The drawing under review shows one solid part. Ordinate dimensions are in mm from its lowest x, y, z. A direction names the side the tool comes from. Give positions to 0.01 mm unless a question says otherwise; leave off trailing zeros. Write each loop counter-clockwise with the first axis right and the second up, starting at its lowest first coordinate (ties: lowest second). Pieces come first, ordered by that corner, then holes. Notation, with made-up numbers: M -14.5,35 L -9.5,35 A29 cw -9.5,62 Z; hole C 71,56.25 d7. An arc over 180 degrees is marked long. One line per item, written item: value. Start each with the question number.
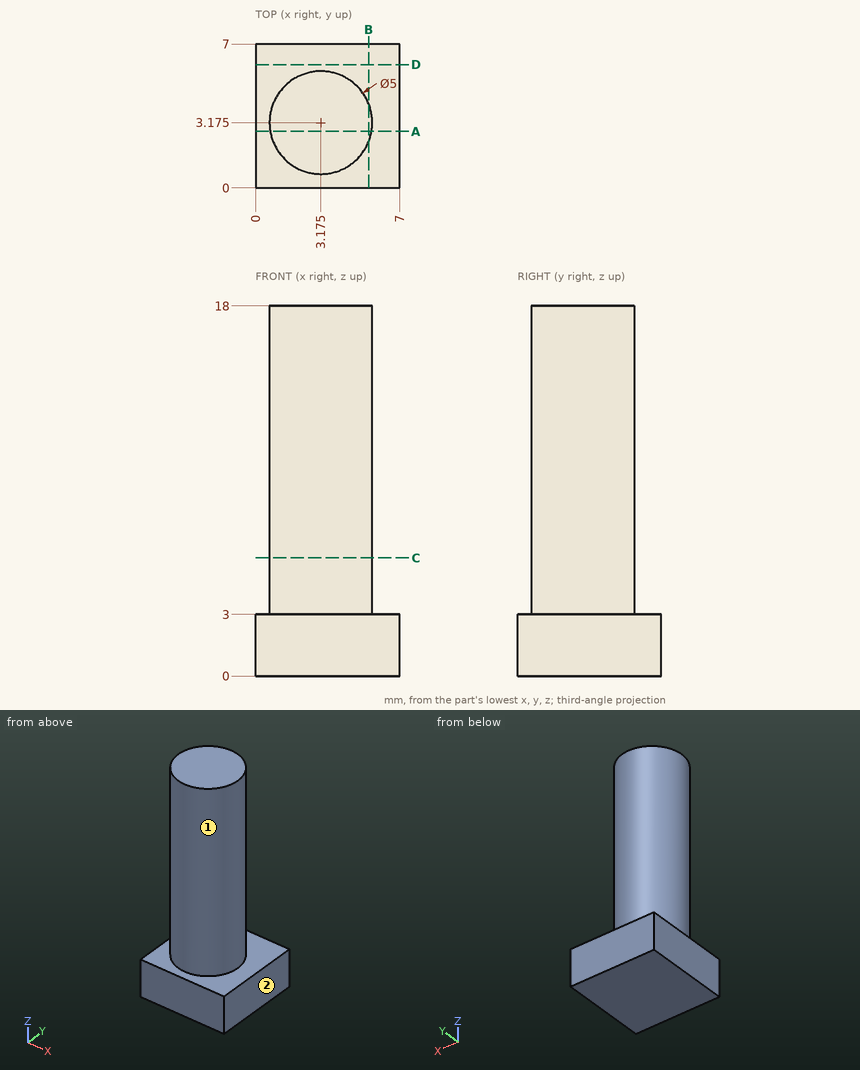
Q1. Take a section at A-A, the plane y = 2.75. Give the boundary of the cut face in (x, z).
Q2. Take a section at B-B, the plane x = 5.5. Give the boundary of the cut face in (y, z), then the cut area to 3 significant figures.
Q3. For P1, Ø2, axis at x = 3, z = 15.5, coming from the -Y side (3 decimals); P2, Ø4, axis at x = 2.5, z = 14.5, coming from the +Y side (3 decimals); P3, Ø4, axis at x = 3, y = 3.5, coming from the -Z side, all flat-tipped, find the tip position at first contact; note any pin that passes through.
Q4. Take a section at D-D, the plane y = 6. Give the boundary of the cut face in (x, z).
Q5. Wall thickness on line 1 (Z direction, x = 0.5, y = 6.5); line 2 (X direction, y = 3.25, z = 5.25); line 3 (Y direction, x = 2.5, z = 8.5): over which ranges is each line inside the solid? List them lowest first. Write a range as from..to.
Q6. Take a section at C-C, the plane z = 5.75. Give the boundary of the cut face in (x, y) (3 decimals), then the cut area to 3 significant figures.
Q7. Machinability: for the marked faces 1 and 2, which of the approach directions +Z, -Z, +X, -X, +Y, -Y give a long, thin tool a straight path to every point of the face, cutting with its end or side? Answer none if there is none.
Results list:
1. outline: M 0,0 L 7,0 L 7,3 L 5.64,3 L 5.64,18 L 0.71,18 L 0.71,3 L 0,3 Z
2. outline: M 0,0 L 7,0 L 7,3 L 4.09,3 L 4.09,18 L 2.26,18 L 2.26,3 L 0,3 Z
2. area: 48.6 mm^2
3. P1: stops at y = 0.675
3. P2: stops at y = 5.675
3. P3: stops at z = 0
4. outline: M 0,0 L 7,0 L 7,3 L 0,3 Z
5. line 1: z = 0..3
5. line 2: x = 0.68..5.67
5. line 3: y = 0.77..5.58
6. outline: C 3.175,3.175 d5
6. area: 19.6 mm^2
7. face 1: +Z
7. face 2: +Z, -Z, +X, +Y, -Y
